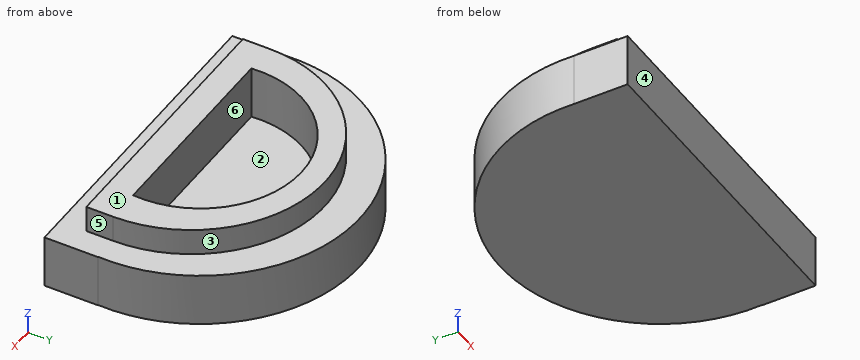
from build123d import *

# Parameters (mm, degrees)
F1_DEPTH = 25.4
F2_W     = 127
F2_H     = 12.7
F3_DEPTH = 12.7
F5_DEPTH = 25.4


with BuildPart() as f1:
    # F0 (on Top) → F1 (new body)
    with BuildSketch(Plane.XY):
        with BuildLine():
            Line((-76.610234, 0), (75.609069, 0))
            ThreePointArc((75.609069, 0), (-0.500583, 79.90958), (-76.610234, 0))
        make_face()
        Polygon((75.789766, 0), (75.609069, 0), (-76.610234, 0), (-76.610234, -25.4), (75.789766, -25.4), align=None)
    extrude(amount=F1_DEPTH)

    # F2 (on face) → F3 (join)
    with BuildSketch(Plane.XY.offset(25.4)):
        with BuildLine():
            Line((-63.5, 0), (63.5, 0))
            ThreePointArc((63.5, 0), (0, 63.5), (-63.5, 0))
        make_face()
        with Locations((0, -6.35)):
            Rectangle(F2_W, F2_H)
    extrude(amount=F3_DEPTH)

    # F4 (on face) → F5 (cut)
    with BuildSketch(Plane.XY.offset(38.1)):
        with BuildLine():
            Line((-48.730817, 0), (47.262773, 0))
            ThreePointArc((47.262773, 0), (-0.734022, 51.986661), (-48.730817, 0))
        make_face()
    extrude(amount=-F5_DEPTH, mode=Mode.SUBTRACT)


solid = f1.part
Check sheet for the modelled part. Datum: model origin and axes. Units: mm. Face numbers are marked on the shaded views. A direction names the side the tool comes from. Give positions to 0.01 mm unless a question says otherwise; leave off trailing zeros. Write each loop counter-clockwise with the first axis right and the second up, starting at its lowest first coordinate (ties: lowest second). Pieces come first, ordered by that corner, then holes. Notation, with made-up numbers: (-12.75, 66) -> (25.25, 66) arc R12 ccw to (25.25, 70) -> close; hole circle Ø9 at (64, 20). An arc over 180 degrees is marked (long way). Write item = value, one per line.
Item 1: Gauge pin test, flat ends, axial feed: pin 1 (6.5 mm diameter, centred on x = -3.5, z = 32, fed in from -Y); pin 2 (1 mm diameter, centred on y = -3.5, z = 28.5, fed in from -X); pin 3 (3 mm diameter, centred on y = 35.5, z = 12.5, fed in from -X). Record the tip position at first contact, or that the pin passes through.
Output:
pin_1 = -12.7
pin_2 = -63.5
pin_3 = -70.42
Item 2: Tool access check on the marked faces 1 and 2. Record the directions out of +Z, -Z, +X, -X, +Y, -Y that give a thin tool (end or side, any length) a straight path to the whole face; none if there is none.
Output:
face_1 = +Z, +X, -X, +Y, -Y
face_2 = +Z
Item 3: Release check for a two-part mould opening along Y. For the marked faces 3, 4, 5 and 6 record: +Y half, -Y half, draft (parallel to the pull), parting line (faces both ways), or undercut.
Output:
face_3 = +Y half
face_4 = -Y half
face_5 = draft
face_6 = undercut
Item 4: Sectioned sample at B-B on y = -4. Record the boundary of the cut face in (x, z).
Output:
outline = (-76.61, 0) -> (75.79, 0) -> (75.79, 25.4) -> (63.5, 25.4) -> (63.5, 38.1) -> (-63.5, 38.1) -> (-63.5, 25.4) -> (-76.61, 25.4) -> close
Item 5: Sectioned sample at D-D on z = 21. Record the boundary of the cut face in (x, y), and give its area (3 significant figures).
Output:
outline = (-76.61, -25.4) -> (75.79, -25.4) -> (75.79, 0) -> (75.61, 0) arc R76.2 ccw (long way) to (-76.61, 0) -> close; hole (-48.73, 0) -> (47.26, 0) arc R48.15 ccw (long way) to start
area = 9,550 mm^2
Item 6: Sectioned sample at C-C on x = 0. Record the boundary of the cut face in (y, z).
Output:
outline = (-25.4, 0) -> (79.91, 0) -> (79.91, 25.4) -> (63.5, 25.4) -> (63.5, 38.1) -> (51.98, 38.1) -> (51.98, 12.7) -> (0, 12.7) -> (0, 38.1) -> (-12.7, 38.1) -> (-12.7, 25.4) -> (-25.4, 25.4) -> close
Item 7: Scan lines: probe 1 along Z at (x, y) = (-40, 51); probe 2 along X at (y, z) = (6.5, 34); probe 3 along Y at (x, z) = (-45, 20.5). Record each from-to range of solid material in increasing order. Write a range as from..to.
Output:
probe_1 = 0..25.4
probe_2 = -63.17..-48.81, 47.34..63.17
probe_3 = -25.4..0, 22.78..65.57
Item 8: Sectioned sample at A-A on z = 33. Record the boundary of the cut face in (x, y), and give its area (3 significant figures).
Output:
outline = (-63.5, -12.7) -> (63.5, -12.7) -> (63.5, 0) arc R63.5 ccw to (-63.5, 0) -> close; hole (-48.73, 0) -> (47.26, 0) arc R48.15 ccw (long way) to start
area = 3,940 mm^2
